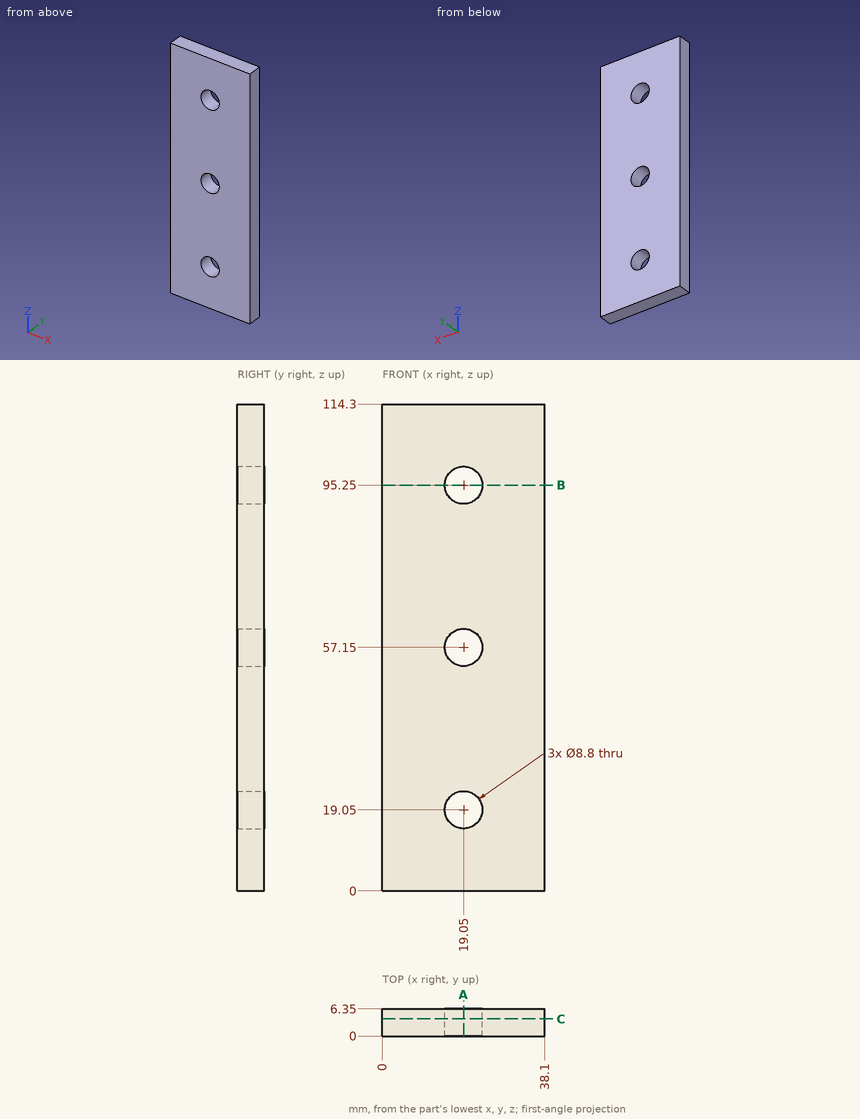
Print and shaded views of the part. All mm, measured from the part's lowest x, y and z. Coordinates: 2 decimals unless noted, no trailing zeros. Order: outer loops, then holes, each group sorted by start corner. A loop starts at its lowest first (then second) coordinate and runs counter-clockwise, first axis right, second up. Notation, with made-up numbers: (36.25, 80.25) - (54.25, 80.25) arc R25 ccw to (54.25, 99.25) - close; hole circle Ø8 at (89.5, 1.25). An arc over 180 degrees is marked (long way). Return JSON: item names as keys, results as strings. Group by question number.
Item 1: Drill centre lines: probe 1 along Z at (x, y) = (19.05, 3.75); probe 2 along Z at (x, y) = (20, 5); probe 3 along X at (y, z) = (6.25, 95). Where is each one in solid material? Low to high. Write a range as from..to.
Item 2: Cut at A-A (x = 19.05). List the corners of the cut face in (y, z).
Item 3: Cut at B-B (z = 95.25). List the corners of the cut face in (x, y), plus the area to 3 significant figures.
Item 4: Cut at C-C (y = 4). List the corners of the cut face in (x, z).
Check values:
{
 "1": {"probe 1": "z = 0..14.65, 23.45..52.75, 61.55..90.85, 99.65..114.3", "probe 2": "z = 0..14.75, 23.35..52.85, 61.45..90.95, 99.55..114.3", "probe 3": "x = 0..14.66, 23.44..38.1"},
 "2": {"outline": "(0, 0) - (6.35, 0) - (6.35, 14.65) - (0, 14.65) - close; (0, 23.45) - (6.35, 23.45) - (6.35, 52.75) - (0, 52.75) - close; (0, 61.55) - (6.35, 61.55) - (6.35, 90.85) - (0, 90.85) - close; (0, 99.65) - (6.35, 99.65) - (6.35, 114.3) - (0, 114.3) - close"},
 "3": {"outline": "(0, 0) - (14.65, 0) - (14.65, 6.35) - (0, 6.35) - close; (23.45, 0) - (38.1, 0) - (38.1, 6.35) - (23.45, 6.35) - close", "area": "186 mm2"},
 "4": {"outline": "(0, 0) - (38.1, 0) - (38.1, 114.3) - (0, 114.3) - close; hole circle Ø8.8 at (19.05, 19.05); hole circle Ø8.8 at (19.05, 57.15); hole circle Ø8.8 at (19.05, 95.25)"}
}
